Here's how the part is built. I have some questions about the finished solid (model axes, mm). A direction names the side the tool comes from. Coordinates: 2 decimals unless noted, no trailing zeros.
Autodesk Fusion 360 part; units mm, degrees
sketch "Sketch1" plane through (0, 0, 0) normal (0, 1, 0) x (1, 0, 0)
  line L0 (31.75, -31.75) -> (-31.75, -31.75)
  line L1 (-31.75, -31.75) -> (-31.75, 31.75)
  line L2 (-31.75, 31.75) -> (31.75, 31.75)
  line L3 (31.75, 31.75) -> (31.75, -31.75)
  line L4 (31.75, -31.75) -> (-31.75, 31.75) construction
  line L5 (-31.75, -31.75) -> (31.75, 31.75) construction
  dimension "d1" = 63.5
  dimension "d2" = 63.5
extrude "Extrude1" add sketch "Sketch1" along normal blind 2.54 makes body 1
sketch "Sketch2" plane through (0, 2.54, 0) normal (0, 1, 0) x (-1, 0, 0)
  line L0 (-31.75, -31.75) -> (31.75, -31.75)
  line L1 (31.75, -31.75) -> (31.75, 31.75)
  line L2 (31.75, 31.75) -> (-31.75, 31.75)
  line L3 (-31.75, 31.75) -> (-31.75, -31.75)
  line L4 (0.635, 31.75) -> (-0.635, 31.75)
  line L5 (-0.635, 31.75) -> (-0.635, -31.75)
  line L6 (-0.635, -31.75) -> (0.635, -31.75)
  line L7 (0.635, -31.75) -> (0.635, 31.75)
  line L8 (0.635, 31.75) -> (-0.635, -31.75) construction
  line L9 (-0.635, 31.75) -> (0.635, -31.75) construction
  dimension "d5" = 1.27
  dimension "d6" = 63.5
ref_plane "WorkPlane1" through (0.635, 0, 0) normal (1, 0, 0) x (0, 1, 0)
sketch "Fin Shape" plane through (0.635, 0, 0) normal (1, 0, 0) x (0, 0, -1)
  line L0 (31.75, 2.54) -> (-31.75, 2.54)
  line L1 (-31.75, 2.54) -> (-31.75, 16.9038)
  line L2 (-31.75, 16.9038) -> (31.75, 16.9038)
  line L3 (31.75, 16.9038) -> (31.75, 2.54)
  line L4 (31.75, 16.9038) -> (-31.75, 19.6763)
  line L5 (-31.75, 19.6763) -> (-31.75, 16.9038)
  dimension "d14" = 63.5
  dimension "d15" = 14.3638
  dimension "d18" = 2.7725
extrude "Extrude3" add sketch "Fin Shape" against normal blind 1.27 separate body makes body 2
pattern_linear "R-Pattern1" count 25 spacing 2.54 along (1, 0, 0) both ways of bodies 2 makes body 3 at (-29.845, 13.04, 10.5833) makes body 4 at (-27.305, 13.04, 10.5833) makes body 5 at (-24.765, 13.04, 10.5833) makes body 6 at (-22.225, 13.04, 10.5833) makes body 7 at (-19.685, 13.04, 10.5833) makes body 8 at (-17.145, 13.04, 10.5833) makes body 9 at (-14.605, 13.04, 10.5833) makes body 10 at (-12.065, 13.04, 10.5833) makes body 11 at (-9.525, 13.04, 10.5833) makes body 12 at (-6.985, 13.04, 10.5833) makes body 13 at (-4.445, 13.04, 10.5833) makes body 14 at (-1.905, 13.04, 10.5833) makes body 15 at (3.175, 13.04, 10.5833) makes body 16 at (5.715, 13.04, 10.5833) makes body 17 at (8.255, 13.04, 10.5833) makes body 18 at (10.795, 13.04, 10.5833) makes body 19 at (13.335, 13.04, 10.5833) makes body 20 at (15.875, 13.04, 10.5833) makes body 21 at (18.415, 13.04, 10.5833) makes body 22 at (20.955, 13.04, 10.5833) makes body 23 at (23.495, 13.04, 10.5833) makes body 24 at (26.035, 13.04, 10.5833) makes body 25 at (28.575, 13.04, 10.5833) makes body 26 at (31.115, 13.04, 10.5833)
combine "Combine2" operation add target body 1 tool bodies 2 4 25 3 26 19 13 10 11 12 17 20 21 7 9 8 24 23 22 6 5 15 14 16 18
equation "d11 = 1.27 * 2 mm"
1. I want a section at A-A (y = 6.5). State how many separate pieces and enclosed holes the cut face has, then the cut area to 3 significant figures.
2. If I drill on line 1 (Y direction, x = -1, z = -8); line 2 (Y direction, x = 25.5, z = -20), over which ranges is the centre line in solid material (lowest first)?
3. On a 3-axis mill with a long thin cutter (end or side, diameter ignored), from which of +Z, -Z, +X, -X, +Y, -Y can I reach the whole of each face in a straight line? I mean faces 4 (the face through (-18.415, 11, 0)), 5 (the face through (0, 0, 0)). Say none if no direction works.
4. For pin 1 Ø5 at (y, z) = (14.5, 4.5) entering from +X (3 decimals); pin 2 Ø2 at (y, z) = (9.5, -11.5) entering from -X (3 decimals); pin 3 Ø0.6 at (x, z) = (-6.5, 8) entering from +Y, each with a flat end and sliding along its axis, tell me the tip position at first contact or that it passes through.
5. Thinking about a two-plate mould opening in X: for faces 1 (the face through (-10.15, 18.27, -0.44)), 2 (the face through (-27.305, 11, 0)), 3 (the face through (-31.115, 11, 0)), which applies, pulls with the +X half, pulls with the -X half, needs draft (parallel to the pull), parting line crosses it, or undercut?
Response values:
1. separate pieces: 25
1. enclosed holes: 0
1. area: 2,020 mm2
2. line 1: y = 0 to 2.54
2. line 2: y = 0 to 17.42
3. face 4: +Z, -Z, +Y
3. face 5: +Z, -Z, +X, -X, -Y
4. pin 1: stops at x = 31.115
4. pin 2: stops at x = -31.115
4. pin 3: stops at y = 2.54
5. face 1: needs draft
5. face 2: undercut
5. face 3: pulls with the -X half
